Geometry: final body of the model. Coordinates: model frame, mm. Face numbers are marked on the shaded views. A direction names the side the tool comes from. Give positions to 0.01 mm unless a question says otherwise; leave off trailing zeros. Order: outer loops, then holes, each group sorted by start corner. A loop starts at its lowest first (then second) coordinate and runs counter-clockwise, first axis right, second up. Notation, with made-up numbers: M 82,-1.75 L 129,-1.75 A12 ccw 129,6.25 Z; hole C -27,-40 d11. An arc over 180 degrees is marked long. One line per item, written item: value. Start each with the question number.
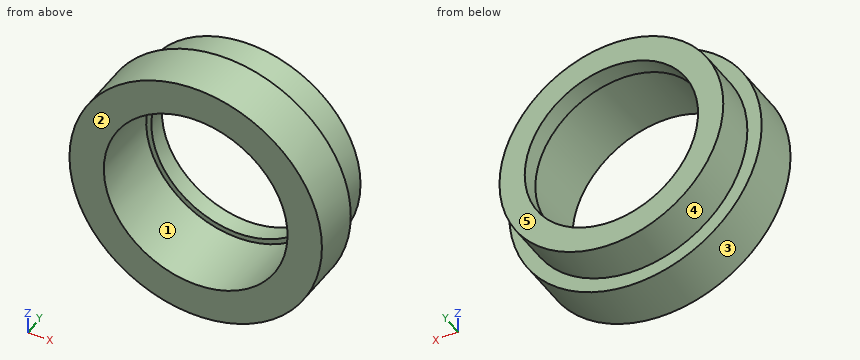
Autodesk Inventor part; units mm, degrees
ref_plane "YZ Plane" through (0, 0, 0) normal (1, 0, 0) x (0, 1, 0)
ref_plane "XZ Plane" through (0, 0, 0) normal (0, 1, 0) x (-1, 0, 0)
ref_plane "XY Plane" through (0, 0, 0) normal (0, 0, 1) x (1, 0, 0)
sketch "Sketch1" plane through (0, 0, 0) normal (0, 1, 0) x (-1, 0, 0)
  circle A0 centre (0, 0) radius 7.5
  dimension "d0" = 15
extrude "Extrusion1" add sketch "Sketch1" along normal blind 3
sketch "Sketch2" plane through (0, 3, 0) normal (0, 1, 0) x (1, 0, 0)
  circle A0 centre (0, 0) radius 7.5
  circle A1 centre (0, 0) radius 6.65
  dimension "d3" = 13.3
extrude "Extrusion2" add sketch "Sketch2" along normal blind 2.5 contours A1
sketch "Sketch3" plane through (0, 5.5, 0) normal (0, 1, 0) x (1, 0, 0)
  circle A0 centre (0, 0) radius 6.65
  circle A1 centre (0, 0) radius 5.15
  dimension "d6" = 10.3
extrude "Extrusion3" cut sketch "Sketch3" against normal through all contours A1
hole "Hole1" at (0, 0, 0) direction (0, 1, 0) diameter 10.917 depth 4.4
properties part number "500-102" material "Steel"
Q1. Section query C-C on y = 3.6. Return loops of the section in (x, z), and give its area (3 significant figures).
Q2. Contact query for a flat-ended pin moving along its axis: pin 1 (1.5 mm diameter, centred on x = 2, z = 1.5, fed in from -Y). Output: stop coordinate, or through.
Q3. Set-up query: the marked faces 4 and 5. Return all of +Z, -Z, +X, -X, +Y, -Y with unobstructed straight access to the full face (end or side cutting, diameter ignored); none if empty.
Q4. Ray query, line 1 along Z through (x, y) = (0, 5.35); line 2 along Z through (x, y) = (0, 2.6). Return the intervals inside material, ascending. Write a range as [from, to].
Q5. Section query D-D on x = -6. Return loops of the section in (y, z).
Q6. Mould query, pull axis Z, two halves, no side actions, for the marked faces 1, 2 and 3. Classes: +Z half, -Z half, draft (parallel to the pull), parting line (faces both ways), or undercut.
Q7. Section query B-B on z = 0. Return loops of the section in (x, y), and give its area (3 significant figures).
Q8. Section query A-A on x = 0. Return loops of the section in (y, z), and give its area (3 significant figures).
Results below:
1. outline: C 0,0 d13.3; hole C 0,0 d10.92
1. area: 45.3 mm2
2. pin 1: through
3. face 4: +Y
3. face 5: +Z, -Z, +X, -X, +Y
4. line 1: [-6.65, -5.15], [5.15, 6.65]
4. line 2: [-7.5, -5.46], [5.46, 7.5]
5. outline: M 0,-4.5 L 3,-4.5 L 3,-2.87 L 5.5,-2.87 L 5.5,2.87 L 3,2.87 L 3,4.5 L 0,4.5 Z
6. face 1: undercut
6. face 2: draft
6. face 3: parting line
7. outline: M -7.5,0 L -5.46,0 L -5.46,4.4 L -5.15,4.4 L -5.15,5.5 L -6.65,5.5 L -6.65,3 L -7.5,3 Z; M 5.15,4.4 L 5.46,4.4 L 5.46,0 L 7.5,0 L 7.5,3 L 6.65,3 L 6.65,5.5 L 5.15,5.5 Z
7. area: 18.9 mm2
8. outline: M 0,-7.5 L 3,-7.5 L 3,-6.65 L 5.5,-6.65 L 5.5,-5.15 L 4.4,-5.15 L 4.4,-5.46 L 0,-5.46 Z; M 0,5.46 L 4.4,5.46 L 4.4,5.15 L 5.5,5.15 L 5.5,6.65 L 3,6.65 L 3,7.5 L 0,7.5 Z
8. area: 18.9 mm2
